Verification items for the finished model (mm, model axes). Face numbers are marked on the shaded views. Give positions to 0.01 mm unless a question says otherwise; leave off trailing zeros. Loops run counter-clockwise (first coordinate to the right, second up) from the corner with the lowest first, then second, coordinate; pieces in that order, holes last. Notation, with made-up numbers: (31, 25) - (73, 25) arc R20 cw to (73, 55) - close; hole circle Ø5 at (64.25, 30.5). An arc over 180 degrees is marked (long way). One line per question, with ' | ' between items. Start each with the question number.
1. Section check D-D, the plane y = 39.5. Enter the section's corners in (x, z), then the cut area to 3 significant figures.
2. Mould release check, pull along X, two halves, no side actions. Record for the marked faces 1, 2 and 3: +X half, -X half, draft (parallel to the pull), parting line (faces both ways), or undercut.
3. Section check B-B, the plane x = 0. Enter the section's corners in (y, z).
4. Section check A-A, the plane y = 77.5. Enter the section's corners in (x, z), then the cut area to 3 significant figures.
5. Thickness scan on line 1 along X through (y, z) = (38.5, 0); line 2 along Z through (x, y) = (-5, 50) (3 decimals); line 3 along X through (y, z) = (61, -7). Record the ranges inside material, lowest first. Write a range as from..to.
6. Depth check by flat-ended pin: pin 1 Ø12 at (y, z) = (62.5, -24) entering from +X; pin 2 Ø1.5 at (x, y) = (-20, 28.5) entering from +Z; pin 3 Ø10 at (x, y) = (10.5, 13.5) entering from +Z; pin 4 Ø7.5 at (x, z) = (-28, 5) entering from -Y. Enter the tip coordinate at first touch or a pass-through.
7. Section check C-C, the plane z = -2. Enter the section's corners in (x, y).
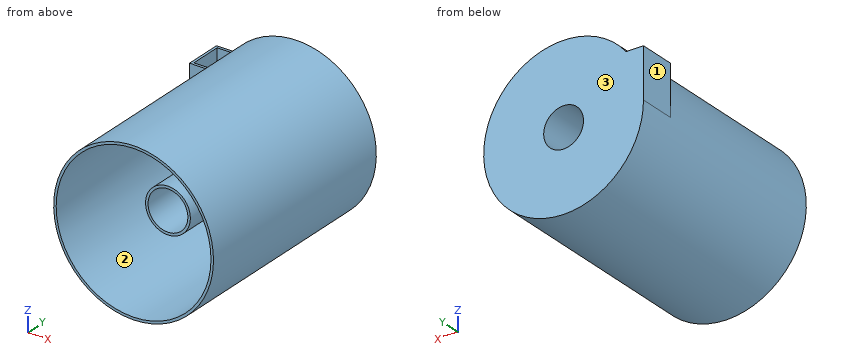
from build123d import *

# Parameters (mm, degrees)
SKETCH_4_W          = 9
SKETCH_4_H          = 14.9
EXTRUDE_3_DEPTH     = 20
SHELL_2_OUTLINE_R   = 31.1
SHELL_2_OUTLINE_R_2 = 9
SHELL_2_DEPTH       = 89
SHELL_2_2_OUTLINE_R = 9
SHELL_2_2_DEPTH     = 19
SHELL_START         = 76.1
SHELL_2_3_DEPTH     = 12.9


# Read off the part's stored shape, not the designer's step: 쉘2
with BuildPart() as part:
    # 스케치3 → 회전1 (revolve)
    with BuildSketch(Plane.XY, mode=Mode.PRIVATE) as revolve_1_sk:
        Polygon((0, 19), (8, 19), (8, 90), (32.1, 90), (32.1, 0), (0, 0), align=None)
    revolve(revolve_1_sk.sketch.rotate(Axis((0, 0, 0), (0, 1, 0)), 90), axis=Axis((0, 0, 0), (0, 1, 0)))

    # 스케치4 → 보스-돌출3 (add)
    with BuildSketch(Plane.XY):
        with Locations((-27.6, 82.55)):
            Rectangle(SKETCH_4_W, SKETCH_4_H)
    extrude(amount=EXTRUDE_3_DEPTH)

    # 쉘2 outline → 쉘2 (cut)
    with BuildSketch(Plane(origin=(0, 0, 0), x_dir=(1, 0, 0), z_dir=(0, 1, 0))):
        Circle(SHELL_2_OUTLINE_R)
        Circle(SHELL_2_OUTLINE_R_2, mode=Mode.SUBTRACT)
    extrude(amount=SHELL_2_DEPTH, mode=Mode.SUBTRACT)

    # Shell 2 2 outline → Shell 2 2 (cut)
    with BuildSketch(Plane(origin=(0, 0, 0), x_dir=(1, 0, 0), z_dir=(0, 1, 0))):
        Circle(SHELL_2_2_OUTLINE_R)
    extrude(amount=SHELL_2_2_DEPTH, mode=Mode.SUBTRACT)

    # Shell 2 3 outline → Shell 2 3 (cut)
    with BuildSketch(Plane(origin=(0, 0, 0), x_dir=(1, 0, 0), z_dir=(0, 1, 0)).offset(SHELL_START)):
        with BuildLine():
            ThreePointArc((-23.816170977, -20), (-29.222362305, -10.642534534), (-31.1, 0))
            Line((-31.1, 0), (-31.1, -20))
            Line((-31.1, -20), (-23.816170977, -20))
        make_face()
    extrude(amount=SHELL_2_3_DEPTH, mode=Mode.SUBTRACT)


solid = part.part
Results list:
1) outline: circle Ø64.2 at (0, 0); circle Ø18 at (0, 0); hole circle Ø62.2 at (0, 0); hole circle Ø16 at (0, 0) | area: 252 mm²
2) face 1: -X half | face 2: undercut | face 3: draft
3) outline: (0, -32.1) - (90, -32.1) - (90, -8) - (19, -8) - (19, -9) - (89, -9) - (89, -31.1) - (0, -31.1) - close; (0, 31.1) - (89, 31.1) - (89, 9) - (19, 9) - (19, 8) - (90, 8) - (90, 32.1) - (0, 32.1) - close
4) outline: (-32.1, 0) arc R32.1 ccw (long way) to (-25.11, 20) - (-23.82, 20) arc R31.1 cw (long way) to (-31.1, 0) - (-31.1, 20) - (-32.1, 20) - close; circle Ø18 at (0, 0); hole circle Ø16 at (0, 0) | area: 250 mm²
5) line 1: -32.1..-31.1, -9..-8, 8..9, 31.1..32.1 | line 2: -31.708..-30.695, -7.483..-6.245, 6.245..7.483, 30.695..31.708 | line 3: -31.33..-30.3, -5.66..-3.87, 3.87..5.66, 30.3..31.33
6) pin 1: x = 26.58 | pin 2: z = 25.69 | pin 3: z = 31.63 | pin 4: y = 0
7) outline: (-32.04, 0) - (-31.04, 0) - (-31.04, 89) - (-8.77, 89) - (-8.77, 19) - (-7.75, 19) - (-7.75, 90) - (-32.04, 90) - close; (7.75, 19) - (8.77, 19) - (8.77, 89) - (31.04, 89) - (31.04, 0) - (32.04, 0) - (32.04, 90) - (7.75, 90) - close
